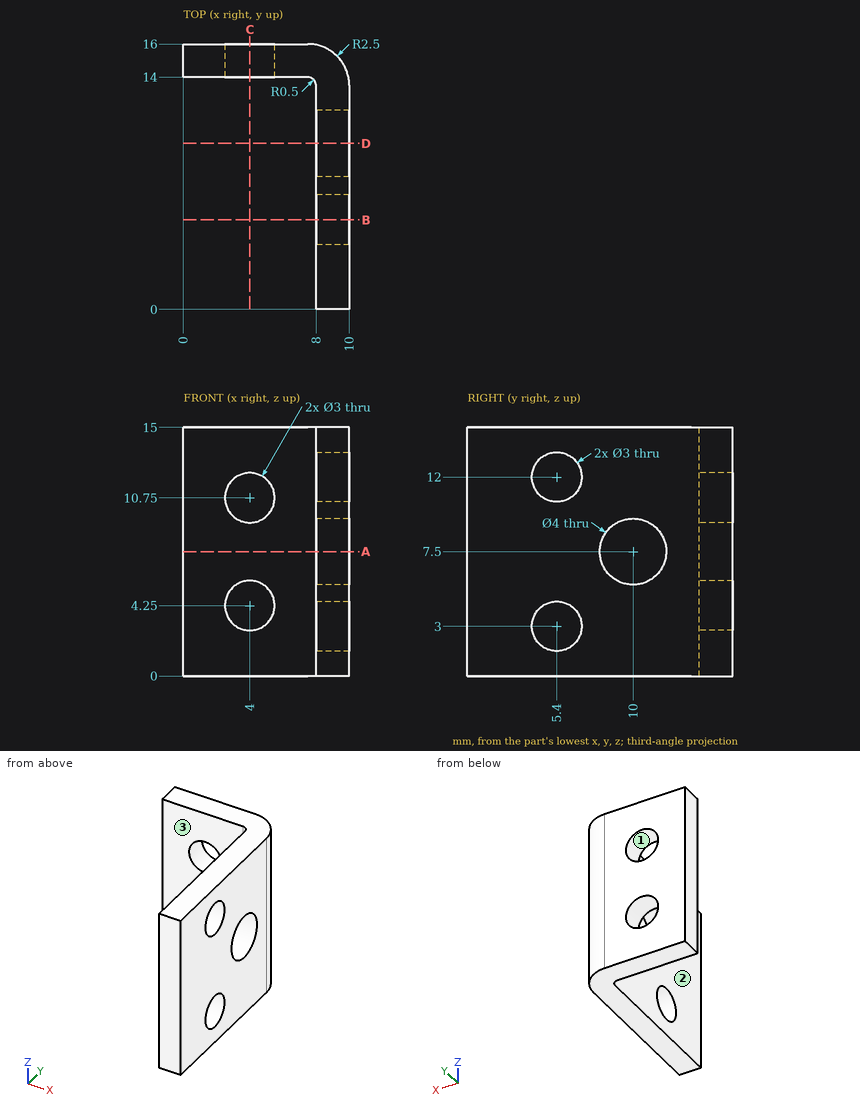
Here's the drawing with two shaded views (mm, measured from the low corner). I have some questions. Round coordinates to 2 decimals unless told otherwise and drop trailing zeros. Order: outer loops, then holes, each group sorted by start corner. A loop starts at its lowest first (then second) coordinate and runs counter-clockwise, first axis right, second up. Notation, with made-up numbers: (7.5, 77.5) -> (54.5, 77.5) arc R25 ccw to (54.5, 114.5) -> close; hole circle Ø3 at (-8, 58). An arc over 180 degrees is marked (long way). Write each question's results on one line, items separated by ' | '. Start each with the question number.
Item 1: If we section it at C-C, the plane x = 4: Write out the boundary of the cut face in (y, z), then the cut area to 3 significant figures.
Item 2: Will these pins go through, and if not, where does the flat tip stop? pin 1 (4 mm diameter, centred on x = 5, z = 9.5, fed in from -Y); pin 2 (7 mm diameter, centred on y = 7, z = 7, fed in from -X).
Item 3: If we section it at B-B, the plane y = 5.4: Write out the boundary of the cut face in (x, z).
Item 4: If we section it at D-D, the plane y = 10: Write out the boundary of the cut face in (x, z), then the cut area to 3 significant figures.
Item 5: Please list where these lines run through material, in increasing order: L1, parallel to Z at x = 4, y = 14.7; L2, parallel to Y at x = 2.25, z = 11.5; L3, parallel to X at y = 8.5, z = 10.
Item 6: If we section it at A-A, the plane z = 7.5: Write out the boundary of the cut face in (x, y).
Item 7: Thinking about a two-plate mould opening in X: for the marked faces 1, 2 and 3, which applies, +X half, -X half, draft (parallel to the pull), parting line (faces both ways), or undercut?
Results:
1) outline: (14, 0) -> (16, 0) -> (16, 2.75) -> (14, 2.75) -> close; (14, 5.75) -> (16, 5.75) -> (16, 9.25) -> (14, 9.25) -> close; (14, 12.25) -> (16, 12.25) -> (16, 15) -> (14, 15) -> close | area: 18.0 mm2
2) pin 1: stops at y = 14 | pin 2: stops at x = 8
3) outline: (8, 0) -> (10, 0) -> (10, 1.5) -> (8, 1.5) -> close; (8, 4.5) -> (10, 4.5) -> (10, 10.5) -> (8, 10.5) -> close; (8, 13.5) -> (10, 13.5) -> (10, 15) -> (8, 15) -> close
4) outline: (8, 0) -> (10, 0) -> (10, 5.5) -> (8, 5.5) -> close; (8, 9.5) -> (10, 9.5) -> (10, 15) -> (8, 15) -> close | area: 22.0 mm2
5) L1: z = 0 to 2.75, 5.75 to 9.25, 12.25 to 15 | L2: y = 14 to 16 | L3: x = 8 to 10
6) outline: (0, 14) -> (7.5, 14) arc R0.5 cw to (8, 13.5) -> (8, 12) -> (10, 12) -> (10, 13.5) arc R2.5 ccw to (7.5, 16) -> (0, 16) -> close; (8, 0) -> (10, 0) -> (10, 8) -> (8, 8) -> close
7) face 1: undercut | face 2: -X half | face 3: draft
